Source: CAD feature listing. Evaluate the final solid. Frame: model axes, mm. Round coordinates to 2 decimals unless told otherwise and drop trailing zeros. Loops run counter-clockwise (first coordinate to the right, second up) from the corner with the lowest first, then second, coordinate; pieces in that order, holes last.
(1) First-contact query: pin 1 Ø3 at (x, y) = (80, -68.5) entering from -Z; pin 2 Ø1 at (x, z) = (-44.5, 2) entering from +Y; pin 3 Ø4 at (x, y) = (32.32, -97.32) entering from -Z; pin 4 Ø1.5 at (x, z) = (-59.5, 2.5) entering from -Y. Flat tips, straight axial feed; report the tip coordinate or a pass-through.
(2) Section B-B, the plane y = 25. Return the cut outline in (x, z) (3 decimals), plus the area to 3 significant figures.
(3) Section C-C, the plane y = -21.5. Return the cut outline in (x, z) (1 decimal), plus the area to 4 significant figures.
(4) Material intervals for probe 1 along X at (y, z) = (88.5, 1.15); probe 2 along Y at (x, z) = (-19, 0.75); probe 3 along Y at (x, z) = (-20.5, 2.65), sorted ascending.
(5) Section A-A, the plane y = -80. Return the cut outline in (x, z) (1 decimal).
(6) Section D-D, the plane x = 18. Return the cut outline in (y, z) (3 decimals).
```python
from build123d import *

# Parameters (mm, degrees)
BOSS_EXTRUDE1_DEPTH = 3.175


with BuildPart() as part:
    # Sketch1 → Boss-Extrude1 (new body)
    with BuildSketch(Plane.XY):
        with BuildLine():
            Line((-38.232117525, -48.334989908), (-60.961358056, -48.334989908))
            ThreePointArc((-60.961358056, -48.334989908), (-64.527927466, -50.321470228), (-64.71669447, -54.399568858))
            ThreePointArc((-64.71669447, -54.399568858), (-45.162805162, -79.848709383), (-17.459350628, -96.051547015))
            ThreePointArc((-17.459350628, -96.051547015), (-16.036418216, -96.080038848), (-14.87146367, -95.262463569))
            ThreePointArc((-14.87146367, -95.262463569), (-8.888558673, -96.210030714), (-13.045252985, -100.616268123))
            ThreePointArc((-13.045252985, -100.616268123), (-45.845334299, -83.275759663), (-68.380015164, -53.801589172))
            ThreePointArc((-68.380015164, -53.801589172), (-65.192805425, 23.622083996), (-36.073719239, 95.431987857))
            ThreePointArc((-36.073719239, 95.431987857), (-35.587957482, 98.278797412), (-37.236596684, 100.64993172))
            Line((-37.236596684, 100.64993172), (-41.103624033, 103.155671407))
            ThreePointArc((-41.103624033, 103.155671407), (-43.974377986, 103.684742176), (-46.378417101, 102.028922117))
            Line((-46.378417101, 102.028922117), (-56.599560294, 86.254961047))
            ThreePointArc((-56.599560294, 86.254961047), (-56.917224028, 84.531308043), (-55.923039481, 83.087879135))
            Line((-55.923039481, 83.087879135), (-55.853863949, 83.043055072))
            ThreePointArc((-55.853863949, 83.043055072), (-54.103522344, 82.73125901), (-52.657612543, 83.765791448))
            ThreePointArc((-52.657612543, 83.765791448), (-48.619561631, 89.956003624), (-44.25417952, 95.919896729))
            ThreePointArc((-44.25417952, 95.919896729), (-44.070317424, 96.300411286), (-44.056473461, 96.722791379))
            ThreePointArc((-44.056473461, 96.722791379), (-41.15632655, 98.522939289), (-42.02094997, 95.220847385))
            ThreePointArc((-42.02094997, 95.220847385), (-42.426877037, 95.079143581), (-42.7383511, 94.782764332))
            ThreePointArc((-42.7383511, 94.782764332), (-47.349935461, 87.504452643), (-51.469836467, 79.936959858))
            ThreePointArc((-51.469836467, 79.936959858), (-57.625378953, 66.65222576), (-62.931273284, 53.005894799))
            Line((-62.931273284, 53.005894799), (-65.323416618, 53.829575804))
            Line((-65.323416618, 53.829575804), (-64.498829719, 56.224350047))
            ThreePointArc((-64.498829719, 56.224350047), (-69.753703666, 53.470378819), (-67.308320476, 48.064996429))
            Line((-67.308320476, 48.064996429), (-66.483733576, 50.459770671))
            Line((-66.483733576, 50.459770671), (-64.091590242, 49.636089666))
            ThreePointArc((-64.091590242, 49.636089666), (-73.69068183, 9.552817578), (-76.050385999, -31.596217123))
            add(Edge.make_bspline(
                [(-76.413674196, -49.035912557), (-76.490697688, -47.59159519), (-76.544524485, -44.699239364), (-76.422918165, -40.352613355), (-76.213699928, -35.991352831), (-76.089673965, -33.05979149), (-76.050385999, -31.596217123)],
                knots=[0.05307402, 0.05307402, 0.05307402, 0.05307402, 0.290327129, 0.527580238, 0.764833347, 1.002086455, 1.002086455, 1.002086455, 1.002086455], degree=3))
            ThreePointArc((-76.413674196, -49.035912557), (-76.449546072, -49.595209625), (-76.264758395, -50.124315962))
            Line((-76.264758395, -50.124315962), (-77.685109529, -50.698175071))
            Line((-77.685109529, -50.698175071), (-78.633899161, -48.349838327))
            ThreePointArc((-78.633899161, -48.349838327), (-80.793035183, -53.875794296), (-75.401231139, -56.350972449))
            Line((-75.401231139, -56.350972449), (-76.350020771, -54.002635705))
            Line((-76.350020771, -54.002635705), (-74.949113638, -53.436632483))
            ThreePointArc((-74.949113638, -53.436632483), (-41.608142422, -93.807518365), (8.312838811, -109.597528539))
            Line((8.312838811, -109.597528539), (8.312838811, -111.108455553))
            Line((8.312838811, -111.108455553), (5.780076045, -111.108455553))
            ThreePointArc((5.780076045, -111.108455553), (10.094826611, -115.180431153), (14.409577176, -111.108455553))
            Line((14.409577176, -111.108455553), (11.876814411, -111.108455553))
            Line((11.876814411, -111.108455553), (11.876814411, -109.597528539))
            ThreePointArc((11.876814411, -109.597528539), (61.797795644, -93.807518365), (95.138766859, -53.436632483))
            Line((95.138766859, -53.436632483), (96.539673992, -54.002635705))
            Line((96.539673992, -54.002635705), (95.590884361, -56.350972449))
            ThreePointArc((95.590884361, -56.350972449), (100.982688404, -53.875794296), (98.823552382, -48.349838327))
            Line((98.823552382, -48.349838327), (97.874762751, -50.698175071))
            Line((97.874762751, -50.698175071), (96.454411616, -50.124315962))
            ThreePointArc((96.454411616, -50.124315962), (96.639199294, -49.595209625), (96.603327418, -49.035912557))
            add(Edge.make_bspline(
                [(96.240039221, -31.596217123), (96.279327187, -33.05979149), (96.40335315, -35.991352831), (96.612571387, -40.352613355), (96.734177707, -44.699239364), (96.68035091, -47.59159519), (96.603327418, -49.035912557)],
                knots=[0.051381708, 0.051381708, 0.051381708, 0.051381708, 0.288634817, 0.525887926, 0.763141035, 1.000394144, 1.000394144, 1.000394144, 1.000394144], degree=3))
            ThreePointArc((96.240039221, -31.596217123), (93.880335052, 9.552817578), (84.281243464, 49.636089666))
            Line((84.281243464, 49.636089666), (86.673386798, 50.459770671))
            Line((86.673386798, 50.459770671), (87.497973697, 48.064996429))
            ThreePointArc((87.497973697, 48.064996429), (89.943356888, 53.470378819), (84.68848294, 56.224350047))
            Line((84.68848294, 56.224350047), (85.513069839, 53.829575804))
            Line((85.513069839, 53.829575804), (83.120926505, 53.005894799))
            ThreePointArc((83.120926505, 53.005894799), (77.815032175, 66.65222576), (71.659489689, 79.936959858))
            ThreePointArc((71.659489689, 79.936959858), (67.539588683, 87.504452643), (62.928004321, 94.782764332))
            ThreePointArc((62.928004321, 94.782764332), (62.616530258, 95.079143581), (62.210603192, 95.220847385))
            ThreePointArc((62.210603192, 95.220847385), (61.345979772, 98.522939289), (64.246126683, 96.722791379))
            ThreePointArc((64.246126683, 96.722791379), (64.259970645, 96.300411286), (64.443832742, 95.919896729))
            ThreePointArc((64.443832742, 95.919896729), (68.809214853, 89.956003624), (72.847265765, 83.765791448))
            ThreePointArc((72.847265765, 83.765791448), (74.293175566, 82.73125901), (76.04351717, 83.043055072))
            Line((76.04351717, 83.043055072), (76.112692703, 83.087879135))
            ThreePointArc((76.112692703, 83.087879135), (77.10687725, 84.531308043), (76.789213515, 86.254961047))
            Line((76.789213515, 86.254961047), (66.568070323, 102.028922117))
            ThreePointArc((66.568070323, 102.028922117), (64.164031207, 103.684742176), (61.293277254, 103.155671407))
            Line((61.293277254, 103.155671407), (57.426249905, 100.64993172))
            ThreePointArc((57.426249905, 100.64993172), (55.777610703, 98.278797412), (56.26337246, 95.431987857))
            ThreePointArc((56.26337246, 95.431987857), (85.382458646, 23.622083996), (88.569668386, -53.801589172))
            ThreePointArc((88.569668386, -53.801589172), (66.03498752, -83.275759663), (33.234906206, -100.616268123))
            ThreePointArc((33.234906206, -100.616268123), (29.078211895, -96.210030714), (35.061116892, -95.262463569))
            ThreePointArc((35.061116892, -95.262463569), (36.226071438, -96.080038848), (37.649003849, -96.051547015))
            ThreePointArc((37.649003849, -96.051547015), (65.352458384, -79.848709383), (84.906347691, -54.399568858))
            ThreePointArc((84.906347691, -54.399568858), (84.717580687, -50.321470228), (81.151011278, -48.334989908))
            Line((81.151011278, -48.334989908), (58.421770747, -48.334989908))
            ThreePointArc((58.421770747, -48.334989908), (10.094826611, -61.266217935), (-38.232117525, -48.334989908))
        make_face()
    extrude(amount=BOSS_EXTRUDE1_DEPTH)


solid = part.part
```
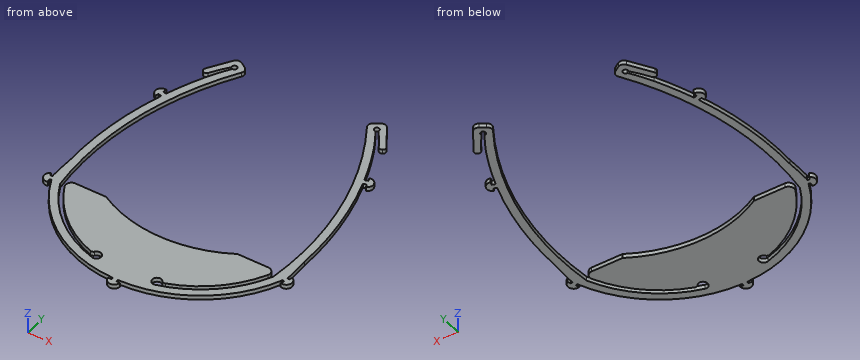
Output values:
1. pin 1: stops at z = 0
1. pin 2: stops at y = 103.68
1. pin 3: passes through
1. pin 4: stops at y = -78.87
2. outline: (-70.88, 0) - (-64.89, 0) - (-64.89, 3.175) - (-70.88, 3.175) - close; (85.08, 0) - (91.07, 0) - (91.07, 3.175) - (85.08, 3.175) - close
2. area: 38.0 mm2
3. outline: (-76.1, 0) - (-70.3, 0) - (-70.3, 3.2) - (-76.1, 3.2) - close; (90.5, 0) - (96.3, 0) - (96.3, 3.2) - (90.5, 3.2) - close
3. area: 37.15 mm2
4. probe 1: x = -55.14 to -49.61, -46.76 to -40.22, 60.41 to 66.95, 69.8 to 75.33
4. probe 2: y = -104.92 to -98.73, -95.5 to -56.79
4. probe 3: y = -104.41 to -98.18, -94.92 to -56.3
5. outline: (-57.7, 0) - (-49.5, 0) - (-49.5, 3.2) - (-57.7, 3.2) - close; (-45, 0) - (65.2, 0) - (65.2, 3.2) - (-45, 3.2) - close; (69.7, 0) - (77.9, 0) - (77.9, 3.2) - (69.7, 3.2) - close
6. outline: (-109.276, 0) - (-60.943, 0) - (-60.943, 3.175) - (-109.276, 3.175) - close
